from build123d import *

# Parameters (mm, degrees)
PAD_DEPTH       = 10
SKETCH001_R     = 3.125
POCKET_DEPTH    = 10.001
SKETCH003_R     = 5.75
POCKET001_DEPTH = 3.5
POCKET002_DEPTH = 5


with BuildPart() as part:
    # Sketch → Pad (new body)
    with BuildSketch(Plane.XY):
        with BuildLine():
            ThreePointArc((-30, 7.5), (-37.5, 0), (-30, -7.5))
            Line((-30, -7.5), (0, -7.5))
            ThreePointArc((0, -7.5), (7.5, 0), (0, 7.5))
            Line((-30, 7.5), (0, 7.5))
        make_face()
    extrude(amount=PAD_DEPTH)

    # Sketch001 → Pocket (cut, through all)
    with BuildSketch(Plane.XY):
        with Locations((-15, 0)):
            Circle(SKETCH001_R)
        Circle(SKETCH001_R)
        with Locations((-30, 0)):
            Circle(SKETCH001_R)
    extrude(amount=POCKET_DEPTH, mode=Mode.SUBTRACT)

    # Sketch003 → Pocket001 (cut)
    with BuildSketch(Plane.XY.offset(10)):
        with Locations((-15, 0)):
            Circle(SKETCH003_R)
        with Locations((-30, 0)):
            Circle(SKETCH003_R)
        Circle(SKETCH003_R)
    extrude(amount=-POCKET001_DEPTH, mode=Mode.SUBTRACT)

    # Sketch004 → Pocket002 (cut)
    with BuildSketch(Plane.XY):
        Polygon((4.979646, -2.875), (4.979646, 2.875), (0, 5.75), (-4.979646, 2.875), (-4.979646, -2.875), (0, -5.75), align=None)
        Polygon((-25.020354, -2.875), (-25.020354, 2.875), (-30, 5.75), (-34.979646, 2.875), (-34.979646, -2.875), (-30, -5.75), align=None)
        Polygon((-10.020354, -2.875), (-10.020354, 2.875), (-15, 5.75), (-19.979646, 2.875), (-19.979646, -2.875), (-15, -5.75), align=None)
    extrude(amount=POCKET002_DEPTH, mode=Mode.SUBTRACT)


solid = part.part
Could you check a few things on this model? Use its own coordinates, in mm. A direction names the side the tool comes from. Coordinates: 2 decimals unless noted, no trailing zeros. Order: outer loops, then holes, each group sorted by start corner. A loop starts at its lowest first (then second) coordinate and runs counter-clockwise, first axis right, second up. Notation, with made-up numbers: (-30, 56.5) -> (0, 56.5) arc R25 ccw to (0, 76.5) -> close; hole circle Ø5 at (63.25, 81). An arc over 180 degrees is marked (long way). One line per item, written item: value. Start each with the question number.
1) Imagine slicing it at C-C on y = 0. Count the separate pieces of the cut face and the enclosed holes in it, plus the area to 3 significant figures.
2) Imagine slicing it at D-D on x = -19. List the corners of the cut face in (y, z) for me, plus the area to 3 significant figures.
3) Imagine slicing it at B-B on z = 1. List the corners of the cut face in (x, y) for me (3 decimals).
4) I'm going to push flat-ended pins straight in: pin 1 (1.5 mm diameter, centred on y = -1, z = 3.5, fed in from +X); pin 2 (5 mm diameter, centred on x = 2, y = -1.5, fed in from -Z); pin 3 (9 mm diameter, centred on x = 0, y = 0, fed in from +Z). Where does each tip first touch, or does it pass through?
5) If I drill on L1, parallel to X at y = 3.5, z = 7.5; L2, parallel to Y at x = -15, z = 5.4 (3 decimals); L3, parallel to X at y = 3, z = 8.75, over which ranges is the centre line in solid material (lowest first)? Write a range as [from, to].
6) Imagine slicing it at A-A on x = -14.5. List the corners of the cut face in (y, z) for me.
7) Which directions (+Z, -Z, +X, -X, +Y, -Y) give clear straight access to the entire face, cutting with the end or side of a thin tool? Please do faces 4 (the cylindrical face through (-20.744, 0.253, 8.274)), 5 (the flat face through (-27.86, -2.48, 5)), 6 (the cylindrical face through (-18.12, 0.14, 5.74)).
8) We'd pull the mould along X, two halves only. Please class faces 1 (the cylindrical face through (-24.516, 1.727, 8.274)), 2 (the cylindrical face through (-37.5, 0.16, 4.93)), 3 (the flat face through (-20.3, 3.4, 10)): +X half, -X half, draft (parallel to the pull), parting line (faces both ways), or undercut.
Answer list:
1. separate pieces: 4
1. enclosed holes: 0
1. area: 152 mm2
2. outline: (-7.5, 0) -> (-3.44, 0) -> (-3.44, 5) -> (3.44, 5) -> (3.44, 0) -> (7.5, 0) -> (7.5, 10) -> (4.13, 10) -> (4.13, 6.5) -> (-4.13, 6.5) -> (-4.13, 10) -> (-7.5, 10) -> close
2. area: 86.7 mm2
3. outline: (-30, -7.5) -> (0, -7.5) arc R7.5 ccw to (0, 7.5) -> (-30, 7.5) arc R7.5 ccw to start; hole (-34.98, -2.875) -> (-30, -5.75) -> (-25.02, -2.875) -> (-25.02, 2.875) -> (-30, 5.75) -> (-34.98, 2.875) -> close; hole (-19.98, -2.875) -> (-15, -5.75) -> (-10.02, -2.875) -> (-10.02, 2.875) -> (-15, 5.75) -> (-19.98, 2.875) -> close; hole (-4.98, -2.875) -> (0, -5.75) -> (4.98, -2.875) -> (4.98, 2.875) -> (0, 5.75) -> (-4.98, 2.875) -> close
4. pin 1: stops at x = 7.5
4. pin 2: stops at z = 5
4. pin 3: stops at z = 6.5
5. L1: x = [-36.63, -34.56], [-25.44, -19.56], [-10.44, -4.56], [4.56, 6.63]
5. L2: y = [-7.5, -3.125], [3.125, 7.5]
5. L3: x = [-36.87, -34.91], [-25.09, -19.91], [-10.09, -4.91], [4.91, 6.87]
6. outline: (-7.5, 0) -> (-5.46, 0) -> (-5.46, 5) -> (-3.08, 5) -> (-3.08, 6.5) -> (-5.73, 6.5) -> (-5.73, 10) -> (-7.5, 10) -> close; (3.08, 5) -> (5.46, 5) -> (5.46, 0) -> (7.5, 0) -> (7.5, 10) -> (5.73, 10) -> (5.73, 6.5) -> (3.08, 6.5) -> close
7. face 4: +Z
7. face 5: -Z
7. face 6: +Z, -Z
8. face 1: undercut
8. face 2: -X half
8. face 3: draft
